Verification items for the finished model (mm, model axes). Face numbers are marked on the shaded views. A direction names the side the tool comes from. Round coordinates to 2 decimals unless told otherwise and drop trailing zeros. Order: outer loops, then holes, each group sorted by start corner. A loop starts at its lowest first (then second) coordinate and runs counter-clockwise, first axis right, second up. Notation, with made-up numbers: (54.5, -20) -> (91.5, -20) arc R18 cw to (91.5, -16) -> close; hole circle Ø9 at (44.25, 48). An arc over 180 degrees is marked (long way). Write item = value, one per line. Start each with the question number.
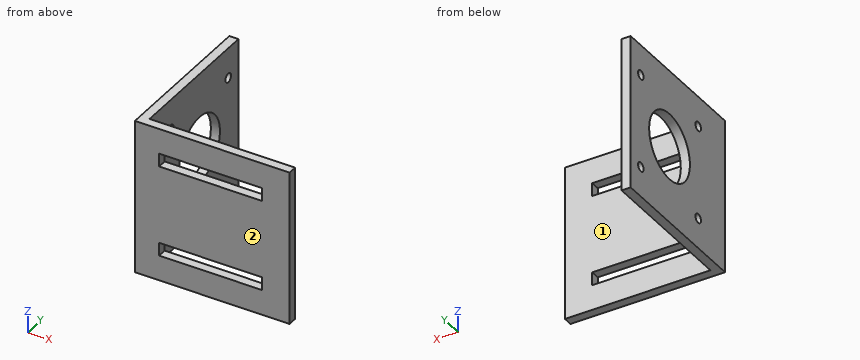
Autodesk Inventor part; units mm, degrees
ref_plane "YZ Plane" through (0, 0, 0) normal (1, 0, 0) x (0, 1, 0)
ref_plane "XZ Plane" through (0, 0, 0) normal (0, 1, 0) x (-1, 0, 0)
ref_plane "XY Plane" through (0, 0, 0) normal (0, 0, 1) x (1, 0, 0)
sketch "Sketch1" plane through (0, 0, 0) normal (0, 0, 1) x (1, 0, 0)
  line L0 (0, 0) -> (0, 51)
  line L1 (0, 51) -> (3, 51)
  line L2 (3, 51) -> (3, 3)
  line L3 (3, 3) -> (51, 3)
  line L4 (51, 3) -> (51, 0)
  line L5 (51, 0) -> (0, 0)
  dimension "d0" = 51
  dimension "d1" = 3
  dimension "d2" = 48
  dimension "d3" = 48
extrude "Extrusion1" add sketch "Sketch1" along normal blind 51
sketch "Sketch2" plane through (3, 3, 0) normal (1, 0, 0) x (0, 0, -1)
  line L0 (0, 48) -> (-51, 48)
  circle A0 centre (-25.5, 27) radius 11
  circle A1 centre (-41, 42.5) radius 1.5
  circle A2 centre (-10, 42.5) radius 1.5
  circle A3 centre (-10, 11.5) radius 1.5
  circle A4 centre (-41, 11.5) radius 1.5
  point P0 (0, -3)
  dimension "d7" = 22
  dimension "d12" = 3
  dimension "d13" = 3
extrude "Extrusion2" cut sketch "Sketch2" against normal up to surface (3 mm away)
sketch "Sketch3" plane through (3, 3, 0) normal (0, 1, 0) x (1, 0, 0)
  line L0 (48, 0) -> (48, -51)
  line L1 (48, -25.5) -> (48, -12.635)
  line L2 (48, -12.635) -> (48, -10.485)
  line L3 (48, -10.485) -> (39, -10.485)
  line L4 (-3, 0) -> (48, 0)
  line L5 (39, 0) -> (39, -7.85)
  line L6 (39, 0) -> (46.85, 0) construction
  line L7 (39, -10.485) -> (39, -8.335)
  line L8 (39, -8.335) -> (5, -8.335)
  line L9 (5, -8.335) -> (5, -12.635)
  line L10 (5, -12.635) -> (39, -12.635)
  line L11 (39, -12.635) -> (39, -10.485)
  line L12 (48, -25.5) -> (-0.1529, -25.5)
  line L13 (39, -40.515) -> (39, -42.665)
  line L14 (39, -42.665) -> (5, -42.665)
  line L15 (5, -42.665) -> (5, -38.365)
  line L16 (5, -38.365) -> (39, -38.365)
  line L17 (39, -38.365) -> (39, -40.515)
  point P0 (39, -43.15)
  dimension "d16" = 12.865
  dimension "d17" = 2.15
  dimension "d18" = 9
  dimension "d20" = 7.85
  dimension "d21" = 270
  dimension "d22" = 2.15
  dimension "d23" = 4.3
extrude "Extrusion3" cut sketch "Sketch3" against normal through all
properties part number "Metal_AttachmentBracket"
(1) Depth check by flat-ended pin: pin 1 (6 mm diameter, centred on y = 22, z = 10.5, fed in from +X). Enter the tip coordinate at first touch or a pass-through.
(2) Set-up check for the marked faces 1 and 2: record each of +Z, -Z, +X, -X, +Y, -Y from which the full face is reachable in a straight line by a thin tool's end or side.
(3) Cross-section at B-B (z = 10). Enter the section's corners in (x, y).
(4) Cross-section at A-A (x = 18.5). Enter the section's corners in (y, z) (3 decimals).
(5) Scan lines: line 1 along Y through (x, z) = (1, 41); line 2 along Y through (x, z) = (1.05, 25.5); line 3 along Z through (x, y) = (1, 14). Record each from-to range of solid material in increasing order. Write a range as from..to.
(6) Cross-section at D-D (y = 30). Enter the section's corners in (x, z).
(7) Cross-section at C-C (y = 14.5). Enter the section's corners in (x, z), and give its area (3 significant figures).
Outcome:
q1.pin_1 = 3
q2.face_1 = +Z, -Z, +X, +Y
q2.face_2 = +Z, -Z, +X, -X, -Y
q3.outline = (0, 0) -> (8, 0) -> (8, 3) -> (3, 3) -> (3, 13) -> (0, 13) -> close; (0, 16) -> (3, 16) -> (3, 44) -> (0, 44) -> close; (0, 47) -> (3, 47) -> (3, 51) -> (0, 51) -> close; (42, 0) -> (51, 0) -> (51, 3) -> (42, 3) -> close
q4.outline = (0, 0) -> (3, 0) -> (3, 8.335) -> (0, 8.335) -> close; (0, 12.635) -> (3, 12.635) -> (3, 38.365) -> (0, 38.365) -> close; (0, 42.665) -> (3, 42.665) -> (3, 51) -> (0, 51) -> close
q5.line_1 = 0..13, 16..44, 47..51
q5.line_2 = 0..19, 41..51
q5.line_3 = 0..8.59, 11.41..39.59, 42.41..51
q6.outline = (0, 0) -> (3, 0) -> (3, 14.5) -> (0, 14.5) -> close; (0, 36.5) -> (3, 36.5) -> (3, 51) -> (0, 51) -> close
q7.outline = (0, 0) -> (3, 0) -> (3, 8.5) -> (0, 8.5) -> close; (0, 11.5) -> (3, 11.5) -> (3, 39.5) -> (0, 39.5) -> close; (0, 42.5) -> (3, 42.5) -> (3, 51) -> (0, 51) -> close
q7.area = 135 mm^2
